Work out the finished part from the listing and answer in its coordinate system (mm). A direction names the side the tool comes from. Round coordinates to 2 decimals unless told otherwise and drop trailing zeros. Write each loop counter-clockwise with the first axis right and the second up, starting at its lowest first coordinate (ties: lowest second). Pieces come first, ordered by that corner, then holes.
1. Determine the mould class of faces 1 (the face through (-26, 2.07, 0.07)), 2 (the face through (-32, -8, 0)), 3 (the face through (32, -6.1, 0)) for opening direction X: pulls with the +X half, pulls with the -X half, needs draft (parallel to the pull), parting line crosses it, or undercut.
2. A tool of negligible diameter and unlimited length cuts with its end or side. For faces 4 (the face through (27.5, -2, 0)), 5 (the face through (24.6, -7.43, -0.07)), 6 (the face through (-27.5, -2, 0)), from which of +Z, -Z, +X, -X, +Y, -Y can it reach the whole face along a straight path? Write none if from no direction.
3. Flat-ended cylindrical pins translate along their axes: pin 1 Ø3 at (x, z) = (-5, 0) entering from -Y; pin 2 Ø3 at (x, z) = (30.5, -0.5) entering from +Y; pin 3 Ø0.8 at (y, z) = (-2.5, -2) entering from -X. Find the tip coordinate at first contact, or state that the pin passes through.
4. Straight lines are drawn through the part: probe 1 along X at (y, z) = (-4.95, 0); probe 2 along X at (y, z) = (-2.5, -2.5); probe 3 along X at (y, z) = (-3.25, 2). For each, find the intervals that lie inside material, in ascending order.
5. Find section D-D (y = 1.5). Write down the section's boundary in (x, z), and give its area (3 significant figures).
6. Find section B-B (x = -32.5). Write down the section's boundary in (y, z), and give its area (3 significant figures).
7. Find section A-A (y = -5). Write down the section's boundary in (x, z).
```python
from build123d import *

# Parameters (mm, degrees)
BOSS_EXTRUDE1_DEPTH = 5
FILLET1_R           = 2
FILLET2_R           = 5
FILLET3_R           = 2
FILLET4_R           = 2
SKETCH3_R           = 3.05
CUT_EXTRUDE1_DEPTH  = 3.1
CHAMFER1_SIZE       = 0.25


with BuildPart() as part:
    # Sketch1 → Boss-Extrude1 (new body, symmetric)
    with BuildSketch(Plane.XY):
        Polygon((-27.5, 3.5), (27.5, 3.5), (27.5, -3), (37.5, -3), (37.5, -8), (27.5, -8), (24, -8), (24, 0), (-24, 0), (-24, -8), (-27.5, -8), (-37.5, -8), (-37.5, -3), (-27.5, -3), align=None)
    extrude(amount=BOSS_EXTRUDE1_DEPTH, both=True)

    # Fillet1
    fillet1_edges = [part.edges().sort_by_distance(p)[0] for p in [
        (24, 0, 0),
        (-24, 0, 0),
    ]]
    fillet(fillet1_edges, radius=FILLET1_R)

    # Fillet2
    fillet2_edges = [part.edges().sort_by_distance(p)[0] for p in [
        (-27.5, 3.5, 0),
        (27.5, 3.5, 0),
    ]]
    fillet(fillet2_edges, radius=FILLET2_R)

    # Fillet3
    fillet3_edges = [part.edges().sort_by_distance(p)[0] for p in [
        (37.5, -5.5, -5),
        (-37.5, -5.5, -5),
        (-37.5, -5.5, 5),
        (37.5, -5.5, 5),
    ]]
    fillet(fillet3_edges, radius=FILLET3_R)

    # Fillet4
    fillet4_edges = [part.edges().sort_by_distance(p)[0] for p in [
        (24, -8, 0),
        (-24, -8, 0),
    ]]
    fillet(fillet4_edges, radius=FILLET4_R)

    # Sketch3 → Cut-Extrude1 (cut)
    with BuildSketch(Plane(origin=(0, -3, 0), x_dir=(1, 0, 0), z_dir=(0, 1, 0))):
        with Locations((32.5, 0)):
            Circle(SKETCH3_R)
        with Locations((-32.5, 0)):
            Circle(SKETCH3_R)
    extrude(amount=-CUT_EXTRUDE1_DEPTH, mode=Mode.SUBTRACT)

    # Chamfer1
    chamfer1_edges = [part.edges().sort_by_distance(p)[0] for p in [
        (29.45, -3, 0),
        (-35.55, -3, 0),
    ]]
    chamfer(chamfer1_edges, length=CHAMFER1_SIZE)


solid = part.part
```
Worked answers:
1. face 1: pulls with the -X half
1. face 2: needs draft
1. face 3: undercut
2. face 4: +Z, -Z, +X, +Y
2. face 5: +Z, -Z, -Y
2. face 6: +Z, -Z, -X, +Y
3. pin 1: stops at y = 0
3. pin 2: stops at y = -3
3. pin 3: stops at x = -27.5
4. probe 1: x = -37.5 to -35.55, -29.45 to -24, 24 to 29.45, 35.55 to 37.5
4. probe 2: x = -27.5 to -24, 24 to 27.5
4. probe 3: x = -37.5 to -34.8, -30.2 to -24, 24 to 30.2, 34.8 to 37.5
5. outline: (-26.5, -5) - (26.5, -5) - (26.5, 5) - (-26.5, 5) - close
5. area: 530 mm2
6. outline: (-8, -5) - (-3, -5) - (-3, -3.3) - (-3.25, -3.05) - (-6.1, -3.05) - (-6.1, 3.05) - (-3.25, 3.05) - (-3, 3.3) - (-3, 5) - (-8, 5) - close
6. area: 31.0 mm2
7. outline: (-37.5, -3) arc R2 ccw to (-35.5, -5) - (-24, -5) - (-24, 5) - (-35.5, 5) arc R2 ccw to (-37.5, 3) - close; (24, -5) - (35.5, -5) arc R2 ccw to (37.5, -3) - (37.5, 3) arc R2 ccw to (35.5, 5) - (24, 5) - close; hole circle Ø6.1 at (-32.5, 0); hole circle Ø6.1 at (32.5, 0)
